For this review, take the finished solid that the model builds, in its own axes (mm). A direction names the side the tool comes from. Round coordinates to 2 decimals unless told otherwise and drop trailing zeros. Order: outer loops, then holes, each group sorted by start corner. A loop starts at its lowest first (then second) coordinate and runs counter-clockwise, first axis right, second up. Notation, with made-up numbers: M 56.25,14 L 109.25,14 A23 ccw 109.25,34 Z; hole C -30,76.5 d3. An arc over 180 degrees is marked long. Answer as a JSON object with one key per item and string values.
from build123d import *

# Parameters (mm, degrees)
F1_DEPTH = 7
F0_R     = 4
F2_DEPTH = 2


with BuildPart() as f1:
    # F0 (on Front) → F1 (new body)
    with BuildSketch(Plane.XZ):
        Polygon((-1.0698140982, 4.0490861801), (-11.6198140982, 4.0490861801), (-14.4198140982, -3.3509138199), (-14.4198140982, -4.9509138199), (-11.6198140982, -12.3509138199), (-1.0698140982, -12.3509138199), (5.3801859018, -7.8009138199), (5.3801859018, -6.9708852422), (5.3801859018, -0.5009138199), align=None)
        Polygon((1.5301859018, -0.6579446913), (1.5301859018, -7.6438829485), (-4.5198140982, -11.1368520771), (-10.5698140982, -7.6438829485), (-10.5698140982, -0.6579446913), (-4.5198140982, 2.8350244373), align=None, mode=Mode.SUBTRACT)
        with BuildLine():
            Line((6.9301859018, -0.5009138199), (5.3801859018, -0.5009138199))
            Line((5.3801859018, -0.5009138199), (5.3801859018, -6.9708852422))
            Line((5.3801859018, -6.9708852422), (6.9301859018, -6.9708852422))
            Line((6.9301859018, -6.9708852422), (10.7727036603, -4.6895619497))
            ThreePointArc((10.7727036603, -4.6895619497), (11.2584820634, -4.2060310818), (11.4565202284, -3.5498575968))
            ThreePointArc((11.4565202284, -3.5498575968), (11.4412037001, -3.3978310982), (11.4094109325, -3.248379192))
            Line((11.4094109325, -3.248379192), (10.6692053247, -3.248379192))
            ThreePointArc((10.6692053247, -3.248379192), (8.1008458295, -4.0583049575), (9.6180241196, -1.8333060186))
            Line((9.6180241196, -1.8333060186), (6.9301859018, -0.5009138199))
        make_face()
        with BuildLine():
            Line((10.679781054, -2.3596310954), (10.1132564961, -2.0787983815))
            ThreePointArc((10.1132564961, -2.0787983815), (10.5230870147, -2.5788610544), (10.6697620079, -3.2085515952))
            ThreePointArc((10.6697620079, -3.2085515952), (10.6696228303, -3.2284673388), (10.6692053247, -3.248379192))
            Line((10.6692053247, -3.248379192), (11.4094109325, -3.248379192))
            ThreePointArc((11.4094109325, -3.248379192), (11.140052623, -2.7256387208), (10.679781054, -2.3596310954))
        make_face()
        with BuildLine():
            Line((10.1132564961, -2.0787983815), (9.6180241196, -1.8333060186))
            ThreePointArc((9.6180241196, -1.8333060186), (8.1008458295, -4.0583049575), (10.6692053247, -3.248379192))
            ThreePointArc((10.6692053247, -3.248379192), (10.6696228303, -3.2284673388), (10.6697620079, -3.2085515952))
            ThreePointArc((10.6697620079, -3.2085515952), (10.5230870147, -2.5788610544), (10.1132564961, -2.0787983815))
        make_face()
    extrude(amount=F1_DEPTH)

    # F0 (on Front) → F2 (join)
    with BuildSketch(Plane.XZ):
        Polygon((-4.5198140982, -11.1368520771), (1.5301859018, -7.6438829485), (1.5301859018, -0.6579446913), (-4.5198140982, 2.8350244373), (-10.5698140982, -0.6579446913), (-10.5698140982, -7.6438829485), align=None)
        with Locations((-4.5198140982, -4.1509138199)):
            Circle(F0_R, mode=Mode.SUBTRACT)
    extrude(amount=F2_DEPTH)


solid = f1.part
1) Add section A-A on x = -2.5. State the section outline as (y, z) points.
Geometry check:
{"outline": "M -7,-12.35 L 0,-12.35 L 0,-7.6 L -2,-7.6 L -2,-9.97 L -7,-9.97 Z; M -7,1.67 L -2,1.67 L -2,-0.7 L 0,-0.7 L 0,4.05 L -7,4.05 Z"}
2) Add section B-B on y = -6. State the section outline as (x, z) points, and give its area (3 significant figures).
Geometry check:
{"outline": "M -14.42,-4.95 L -11.62,-12.35 L -1.07,-12.35 L 5.38,-7.8 L 5.38,-6.97 L 6.93,-6.97 L 10.77,-4.69 A1.4 ccw 11.46,-3.55 A1.4 ccw 10.68,-2.36 L 6.93,-0.5 L 5.38,-0.5 L -1.07,4.05 L -11.62,4.05 L -14.42,-3.35 Z; hole M -10.57,-7.64 L -4.52,-11.14 L 1.53,-7.64 L 1.53,-0.66 L -4.52,2.84 L -10.57,-0.66 Z", "area": "176 mm²"}
3) Insertion check: P1, Ø2, axis at x = -1, z = -1.5, coming from the +Y side; P2, Ø1.7, axis at x = 6, y = -2, coming from the -Z side; P3, Ø0.9, axis at y = -2.5, z = -7.5, coming from the +X side; P4, Ø7, axis at x = -4.52, z = -4.15, coming from the +Y side. Each pin has a flat end and moves straight along its axis. Give the tip position at first contact, or say it passes through.
Geometry check:
{"P1": "stops at y = 0", "P2": "stops at z = -7.96", "P3": "stops at x = 5.38", "P4": "passes through"}
4) For L1, parallel to Z at x = 6.75, y = -6; L2, parallel to X at y = -6.5, z = 1.25; L3, parallel to X at y = -4.75, z = -3, list the stretches that pass through material, from the lowest coordinate up.
Geometry check:
{"L1": "z = -6.97 to -0.5", "L2": "x = -12.68 to -7.27, -1.77 to 2.9", "L3": "x = -14.29 to -10.57, 1.53 to 11.32"}
5) Add section D-D on x = 0.5. State the section outline as (y, z) points.
Geometry check:
{"outline": "M -7,-11.24 L 0,-11.24 L 0,2.94 L -7,2.94 L -7,-0.06 L -2,-0.06 L -2,-8.24 L -7,-8.24 Z"}
6) Machinability: for faces 1 (the flat face through (-9, -2, -4)), 2 (the flat face through (6, -3, -0.501)), 3 (the flat face through (5.38, -3.5, -7.4)), 4 (the flat face through (-14.42, -3, -4)), 5 (the flat face through (-6, -3, 4.049)), which of the approach directions +Z, -Z, +X, -X, +Y, -Y give a long, thin tool a straight path to every point of the face, cutting with its end or side? Answer none if there is none.
Geometry check:
{"face 1": "-Y", "face 2": "+Z, +X, +Y, -Y", "face 3": "-Z, +X, +Y, -Y", "face 4": "+Z, -Z, -X, +Y, -Y", "face 5": "+Z, +X, -X, +Y, -Y"}
7) Add section C-C on z = 1. State the section outline as (x, y) points.
Geometry check:
{"outline": "M -12.77,-7 L -7.7,-7 L -7.7,-2 L -1.34,-2 L -1.34,-7 L 3.25,-7 L 3.25,0 L -12.77,0 Z"}
8) Mouldability with a two-part tool opening along Z and no side actions: class faces 6 (the flat face through (6, -3, -6.971)), 7 (the flat face through (2.2, -3.451, 1.742)), 8 (the cylindrical face through (-8.516, -0.986, -3.975)) as +Z half, -Z half, draft (parallel to the pull), parting line (faces both ways), or undercut.
Geometry check:
{"face 6": "-Z half", "face 7": "+Z half", "face 8": "undercut"}
